Could you check a few things on this drawing? It's one solid part, dimensions in mm from its lowest x, y, z. Coordinates: 2 decimals unless noted, no trailing zeros. Order: outer loops, then holes, each group sorted by start corner. A loop starts at its lowest first (then second) coordinate and runs counter-clockwise, first axis right, second up. Notation, with made-up numbers: (19.25, 1) -> (34.25, 1) arc R17 cw to (34.25, 33) -> close; hole circle Ø3 at (-22.75, 12). An arc over 180 degrees is marked (long way). Use a Markdown table: item, result. Add a question column.
1. If I drill on line 1 along Z through (x, y) = (57.5, 0.65); line 2 along X through (y, z) = (0.45, 64); line 3 along X through (y, z) = (0.8, 100.5), over which ranges is the centre line in solid material (lowest first)? Write a range as from..to.
2. Suppose I cut it at A-A, the plane z = 64. List the corners of the cut face in (x, y) for me.
3. Suppose I cut it at C-C, the plane y = 0.8. State how many separate pieces and enclosed holes the cut face has, then the cut area to 3 significant figures.
4. Suppose I cut it at D-D, the plane x = 50. List the corners of the cut face in (y, z) for me.
5. Suppose I cut it at B-B, the plane x = 2.5. List the corners of the cut face in (y, z) for me, then the cut area to 3 significant figures.
6. For pin 1 Ø0.5 at (x, y) = (56, 1) entering from +Z; pin 2 Ø0.8 at (y, z) = (0.5, 103) entering from -X, each with a flat end and sliding along its axis, tell me the tip position at first contact or that it passes through.
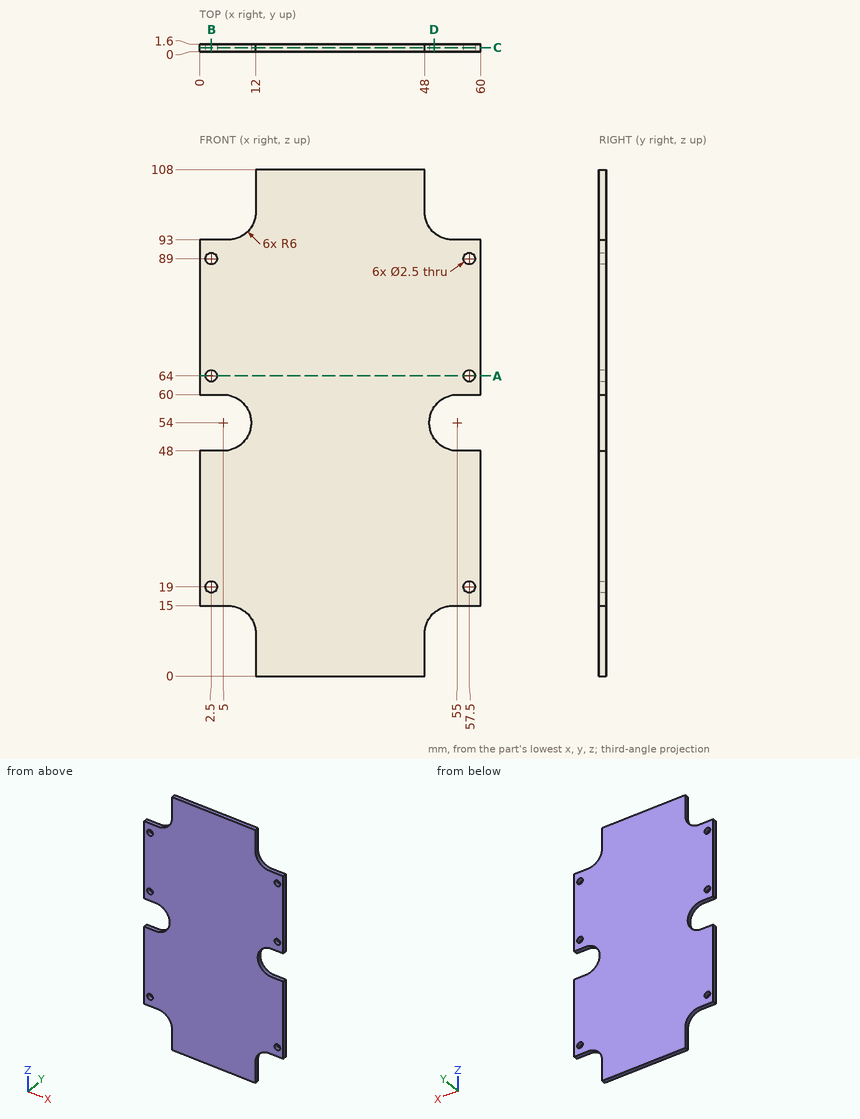
Worked out:
| question | item | result |
|---|---|---|
| 1 | line 1 | z = 15..17.75, 20.25..48, 60..62.75, 65.25..87.75, 90.25..93 |
| 1 | line 2 | x = 0..1.25, 3.75..56.25, 58.75..60 |
| 1 | line 3 | x = 12..48 |
| 2 | outline | (0, 0) -> (1.25, 0) -> (1.25, 1.6) -> (0, 1.6) -> close; (3.75, 0) -> (56.25, 0) -> (56.25, 1.6) -> (3.75, 1.6) -> close; (58.75, 0) -> (60, 0) -> (60, 1.6) -> (58.75, 1.6) -> close |
| 3 | separate pieces | 1 |
| 3 | enclosed holes | 6 |
| 3 | area | 5,530 mm² |
| 4 | outline | (0, 13.47) -> (1.6, 13.47) -> (1.6, 50.68) -> (0, 50.68) -> close; (0, 57.32) -> (1.6, 57.32) -> (1.6, 94.53) -> (0, 94.53) -> close |
| 5 | outline | (0, 15) -> (1.6, 15) -> (1.6, 17.75) -> (0, 17.75) -> close; (0, 20.25) -> (1.6, 20.25) -> (1.6, 48) -> (0, 48) -> close; (0, 60) -> (1.6, 60) -> (1.6, 62.75) -> (0, 62.75) -> close; (0, 65.25) -> (1.6, 65.25) -> (1.6, 87.75) -> (0, 87.75) -> close; (0, 90.25) -> (1.6, 90.25) -> (1.6, 93) -> (0, 93) -> close |
| 5 | area | 93.6 mm² |
| 6 | pin 1 | stops at z = 93 |
| 6 | pin 2 | stops at x = 12 |
